Design review of the part built by this model. Coordinates are the model's own, in mm. Face numbers are marked on the shaded views. Coordinates: 2 decimals unless noted, no trailing zeros. Write each loop counter-clockwise with the first axis right and the second up, starting at its lowest first coordinate (ties: lowest second). Pieces come first, ordered by that corner, then holes.
Q1. Take a section at D-D (x = -8). Give the boundary of the cut face in (y, z), and give its area (3 significant figures).
Q2. Take a section at A-A (y = 20.5). State how many separate pieces and enclosed holes the cut face has, and give its area (3 significant figures).
Q3. Insertion check: pin 1 (0.9 mm diameter, centred on x = -0.5, z = 41.5, fed in from +Y); pin 2 (1.5 mm diameter, centred on y = 3.5, z = -34.5, fed in from -X); pin 3 (6 mm diameter, centred on y = 27, z = -34, fed in from -X); pin 4 (12 mm diameter, centred on y = 18, z = 13.5, fed in from +X). Each pin has a flat end and moves straight along its axis. Give the tip position at first contact, or say it passes through.
Q4. Take a section at B-B (y = 33.5). Give the boundary of the cut face in (x, z).
Q5. Mouldability with a two-part tool opening along X and no side actions: class the marked faces 1, 2 and 3 as pulls with the +X half, pulls with the -X half, needs draft (parallel to the pull), parting line crosses it, or undercut.
Q6. Take a section at C-C (x = 36). Give the boundary of the cut face in (y, z), and give its area (3 significant figures).
Q7. For probe 1 along X at (y, z) = (29, 0); probe 2 along Z at (x, y) = (29, 23.25); probe 3 along Z at (x, y) = (-11.5, 4.5), list the stretches that pass through material, from the lowest coordinate up.
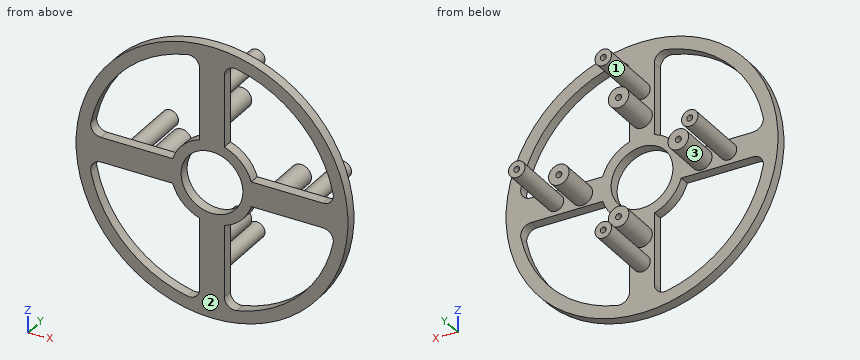
```python
from build123d import *

# Parameters (mm, degrees)
SKETCH1_R           = 66
BOSS_EXTRUDE1_DEPTH = 5
FILLET1_R           = 5
SKETCH3_R           = 5
BOSS_EXTRUDE3_DEPTH = 19.5
SKETCH4_R           = 20
BOSS_EXTRUDE4_DEPTH = 5
CIRPATTERN1_COUNT   = 4
SKETCH5_R           = 15
CUT_EXTRUDE1_DEPTH  = 10
SKETCH6_R           = 4
BOSS_EXTRUDE5_DEPTH = 32.25
CIRPATTERN2_COUNT   = 4
CUT_EXTRUDE3_START  = -6
SKETCH7_R           = 1.45
CUT_EXTRUDE3_DEPTH  = 103.5
CIRPATTERN3_COUNT   = 4


with BuildPart() as part:
    # Sketch1 → Boss-Extrude1 (new body)
    with BuildSketch(Plane(origin=(0, 0, 0), x_dir=(1, 0, 0), z_dir=(0, 1, 0))):
        with Locations(Location((0, 0, 0), (0, 0, 270))):
            Circle(SKETCH1_R)
        with BuildLine():
            Line((-6, -59.699246226), (-6, -6))
            Line((-6, -6), (-59.699246226, -6))
            ThreePointArc((-59.699246226, -6), (-42.426406871, -42.426406871), (-6, -59.699246226))
        make_face(mode=Mode.SUBTRACT)
        with BuildLine():
            Line((6, -59.699246226), (6, -6))
            Line((6, -6), (59.699246226, -6))
            ThreePointArc((59.699246226, -6), (42.426406871, -42.426406871), (6, -59.699246226))
        make_face(mode=Mode.SUBTRACT)
        with BuildLine():
            Line((-59.699246226, 6), (-6, 6))
            Line((-6, 6), (-6, 59.699246226))
            ThreePointArc((-6, 59.699246226), (-42.426406871, 42.426406871), (-59.699246226, 6))
        make_face(mode=Mode.SUBTRACT)
        with BuildLine():
            Line((6, 6), (6, 59.699246226))
            ThreePointArc((6, 59.699246226), (42.426406871, 42.426406871), (59.699246226, 6))
            Line((59.699246226, 6), (6, 6))
        make_face(mode=Mode.SUBTRACT)
    extrude(amount=BOSS_EXTRUDE1_DEPTH)

    # Fillet1
    fillet1_edges = [part.edges().sort_by_distance(p)[0] for p in [
        (-6, 2.5, -59.699246226),
        (-59.699246226, 2.5, -6),
        (-6, 2.5, -6),
        (6, 2.5, 59.699246226),
        (59.699246226, 2.5, 6),
        (6, 2.5, 6),
        (59.699246226, 2.5, -6),
        (6, 2.5, -59.699246226),
        (6, 2.5, -6),
        (-59.699246226, 2.5, 6),
        (-6, 2.5, 59.699246226),
        (-6, 2.5, 6),
    ]]
    fillet(fillet1_edges, radius=FILLET1_R)

    # Sketch3 → Boss-Extrude3 (add)
    with BuildSketch(Plane(origin=(0, 5, 0), x_dir=(1, 0, 0), z_dir=(0, 1, 0))):
        with Locations(Location((-29, 0, 0), (0, 0, 270))):
            Circle(SKETCH3_R)
    boss_extrude3 = extrude(amount=BOSS_EXTRUDE3_DEPTH)

    # Sketch4 → Boss-Extrude4 (add)
    with BuildSketch(Plane(origin=(0, 5, 0), x_dir=(1, 0, 0), z_dir=(0, 1, 0))):
        Circle(SKETCH4_R)
    extrude(amount=-BOSS_EXTRUDE4_DEPTH)

    # CirPattern1: Boss-Extrude3 ×4 about axis
    cirpattern1_axis = Axis((0, 0, 0), (0, 1, 0))
    for i in range(1, CIRPATTERN1_COUNT):
        add(boss_extrude3.rotate(cirpattern1_axis, i * 360 / CIRPATTERN1_COUNT))

    # Sketch5 → Cut-Extrude1 (cut)
    with BuildSketch(Plane(origin=(0, 5, 0), x_dir=(1, 0, 0), z_dir=(0, 1, 0))):
        with Locations(Location((0, 0, 0), (0, 0, 270))):
            Circle(SKETCH5_R)
    extrude(amount=-CUT_EXTRUDE1_DEPTH, mode=Mode.SUBTRACT)

    # Sketch6 → Boss-Extrude5 (add)
    with BuildSketch(Plane(origin=(0, 5, 0), x_dir=(1, 0, 0), z_dir=(0, 1, 0))):
        with Locations(Location((-42, 0, 0), (0, 0, 270))):
            Circle(SKETCH6_R)
    boss_extrude5 = extrude(amount=BOSS_EXTRUDE5_DEPTH)

    # CirPattern2: Boss-Extrude5 ×4 about axis
    cirpattern2_axis = Axis((0, 0, 0), (0, 1, 0))
    for i in range(1, CIRPATTERN2_COUNT):
        add(boss_extrude5.rotate(cirpattern2_axis, i * 360 / CIRPATTERN2_COUNT))

    # Sketch7 → Cut-Extrude3 (cut)
    with BuildSketch(Plane(origin=(0, 24.5, 0), x_dir=(1, 0, 0), z_dir=(0, 1, 0)).offset(CUT_EXTRUDE3_START)):
        with Locations(Location((-29, 0, 0), (0, 0, 270))):
            Circle(SKETCH7_R)
        with Locations(Location((-42, 0, 0), (0, 0, 270))):
            Circle(SKETCH7_R)
    cut_extrude3 = extrude(amount=CUT_EXTRUDE3_DEPTH, mode=Mode.SUBTRACT)

    # CirPattern3: Cut-Extrude3 ×4 about axis
    cirpattern3_axis = Axis((0, 0, 0), (0, 1, 0))
    for i in range(1, CIRPATTERN3_COUNT):
        add(cut_extrude3.rotate(cirpattern3_axis, i * 360 / CIRPATTERN3_COUNT), mode=Mode.SUBTRACT)


solid = part.part
```
Response:
1. outline: (0, -65.51) - (5, -65.51) - (5, -57.89) - (0, -57.89) - close; (0, -18.33) - (5, -18.33) - (5, -12.69) - (0, -12.69) - close; (0, 12.69) - (5, 12.69) - (5, 18.33) - (0, 18.33) - close; (0, 57.89) - (5, 57.89) - (5, 65.51) - (0, 65.51) - close
1. area: 133 mm2
2. separate pieces: 8
2. enclosed holes: 8
2. area: 462 mm2
3. pin 1: stops at y = 18.5
3. pin 2: stops at x = -56.72
3. pin 3: stops at x = -3.72
3. pin 4: passes through
4. outline: circle Ø8 at (-42, 0); circle Ø8 at (0, -42); circle Ø8 at (0, 42); circle Ø8 at (42, 0); hole circle Ø2.9 at (-42, 0); hole circle Ø2.9 at (0, -42); hole circle Ø2.9 at (0, 42); hole circle Ø2.9 at (42, 0)
5. face 1: parting line crosses it
5. face 2: needs draft
5. face 3: undercut
6. outline: (0, -55.32) - (5, -55.32) - (5, -48) - (0, -48) - close; (0, -6) - (5, -6) - (5, 6) - (0, 6) - close; (0, 48) - (5, 48) - (5, 55.32) - (0, 55.32) - close
6. area: 133 mm2
7. probe 1: x = -46 to -43.45, -40.55 to -38, 38 to 40.55, 43.45 to 46
7. probe 2: z = -5 to -1.45, 1.45 to 5
7. probe 3: z = -64.99 to -58.86, -16.36 to -9.63, 9.63 to 16.36, 58.86 to 64.99
